Autodesk Inventor part; units mm, degrees
ref_plane "YZ Plane" through (0, 0, 0) normal (1, 0, 0) x (0, 1, 0)
ref_plane "XZ Plane" through (0, 0, 0) normal (0, 1, 0) x (-1, 0, 0)
ref_plane "XY Plane" through (0, 0, 0) normal (0, 0, 1) x (1, 0, 0)
sketch "Sketch1" plane through (0, 0, 0) normal (0, 0, 1) x (1, 0, 0)
  circle A0 centre (130.9, -80) radius 15 construction
  line L0 (0, 0) -> (117.2543, 0) construction
  line L1 (-60.9, -65.8) -> (60.9, -65.8)
  line L2 (60.9, -94.2) -> (60.9, -65.8)
  line L3 (60.9, -94.2) -> (-60.9, -94.2)
  line L4 (-60.9, -65.8) -> (-60.9, -94.2)
  circle A1 centre (130.9, -80) radius 15.3
  circle A2 centre (130.9, -80) radius 17.3
  circle A3 centre (112.1, -80) radius 1.5
  circle A4 centre (112.1, -80) radius 3.5
  line L5 (109.5309, -77.6231) -> (118.2011, -68.2515)
  line L6 (109.5309, -82.3769) -> (118.2011, -91.7485)
  circle A5 centre (-45.9, -80) radius 3.15
  circle A6 centre (45.9, -80) radius 3.15
  point P0 (60.9, -80)
  dimension "d0" = 30
  dimension "d1" = 70
  dimension "d2" = 0.3
  dimension "d3" = 2
  dimension "d4" = 3
  dimension "d6" = 2
extrude "Extrusion1" add sketch "Sketch1" against normal blind 10 contours A4 A2 | A4 A2 | A4 L5 A2 | A2 A4 | A2 L6 A4
pattern_circular "Circular Pattern1" count 3 over 360 about axis through (130.9, -80, 0) along (0, 0, -1) of "Extrusion1"
properties part number "Chamber Holder"
Can you work these out from the model? Positions are in its coordinate system, mm. Give positions to 0.01 mm unless a question says otherwise; leave off trailing zeros. Order: outer loops, then holes, each group sorted by start corner. A loop starts at its lowest first (then second) coordinate and runs counter-clockwise, first axis right, second up. Notation, with made-up numbers: M -22,-38 L 9,-38 A23 ccw 9,-2 Z; hole C -21,67 d6. An arc over 180 degrees is marked long. One line per item, written item: value.
Item 1: If we section it at A-A on x = 117: Write out the boundary of the cut face in (y, z).
Verdict:
outline: M -90.45,-10 L -86.39,-10 L -86.39,0 L -90.45,0 Z; M -73.61,-10 L -69.55,-10 L -69.55,0 L -73.61,0 Z
Item 2: For pin 1 (1.5 mm diameter, centred on x = 118, z = -4, fed in from -Y); pin 2 (4 mm diameter, centred on x = 125.5, z = -3, fed in from +Y); pin 3 (2 mm diameter, centred on x = 122, z = -5, fed in from -Y), each with a flat end and sliding along its axis, tell me the tip position at first contact or that it passes through.
Verdict:
pin 1: y = -92.32
pin 2: y = -63.03
pin 3: y = -95.39
Item 3: If we section it at B-B on y = -80: Write out the boundary of the cut face in (x, z), and give its area (3 significant figures).
Verdict:
outline: M 108.6,-10 L 110.6,-10 L 110.6,0 L 108.6,0 Z; M 113.6,-10 L 115.6,-10 L 115.6,0 L 113.6,0 Z; M 146.2,-10 L 148.2,-10 L 148.2,0 L 146.2,0 Z
area: 60.0 mm2
Item 4: If we mould it in two halves opening along Y, with no side actions, what happens to faces 1 (the face through (121, -68, -10)), 2 (the face through (113.53, -79.55, -4.93)), 3 (the face through (142.082, -60.706, -4.93))? For each: pulls with the +Y half, pulls with the -Y half, needs draft (parallel to the pull), parting line crosses it, or undercut.
Verdict:
face 1: needs draft
face 2: undercut
face 3: pulls with the +Y half
Item 5: Please list where these lines run through material, in increasing order: line 1 (X direction, y = -80, z = -5); line 2 (X direction, y = -81, z = -5); line 3 (Y direction, x = 140.3, z = -3.5).
Verdict:
line 1: 108.6 to 110.6, 113.6 to 115.6, 146.2 to 148.2
line 2: 108.75 to 110.98, 113.22 to 115.63, 146.17 to 148.17
line 3: -99.78 to -97.78, -94.78 to -92.07, -67.93 to -65.22, -62.22 to -60.22
Item 6: If we section it at D-D on y = -69: Write out the boundary of the cut face in (x, z), and give its area (3 significant figures).
Verdict:
outline: M 117.51,-10 L 120.27,-10 L 120.27,0 L 117.51,0 Z; M 141.53,-10 L 145.6,-10 L 145.6,0 L 141.53,0 Z
area: 68.2 mm2
